```python
from build123d import *

# Parameters (mm, degrees)
SKETCH1_W           = 64
SKETCH1_H           = 42
BOSS_EXTRUDE1_DEPTH = 14.5
FILLET1_R           = 8
FILLET2_R           = 2
SHELL1_T            = -1.6
CUT_EXTRUDE1_REACH  = 70.9
SKETCH2_W           = 3.8
SKETCH2_H           = 24.8
SKETCH3_R           = 3
BOSS_EXTRUDE2_DEPTH = 7.000000018
CUT_EXTRUDE2_REACH  = 77.447
SKETCH4_R           = 1.6
SKETCH5_R           = 4
CUT_EXTRUDE3_DEPTH  = 0.6


with BuildPart() as part:
    # Sketch1 → Boss-Extrude1 (new body)
    with BuildSketch(Plane.XY):
        Rectangle(SKETCH1_W, SKETCH1_H)
    extrude(amount=BOSS_EXTRUDE1_DEPTH)

    # Fillet1
    fillet1_edges = [part.edges().sort_by_distance(p)[0] for p in [
        (-32, 21, 7.25),
        (32, 21, 7.25),
        (32, -21, 7.25),
        (-32, -21, 7.25),
    ]]
    fillet(fillet1_edges, radius=FILLET1_R)

    # Fillet2
    fillet2_edges = [part.edges().sort_by_distance(p)[0] for p in [
        (0, -21, 14.5),
        (-32, 0, 14.5),
        (32, 0, 14.5),
        (0, 21, 14.5),
        (29.656854249, 18.656854249, 14.5),
        (-29.656854249, 18.656854249, 14.5),
        (29.656854249, -18.656854249, 14.5),
        (-29.656854249, -18.656854249, 14.5),
    ]]
    fillet(fillet2_edges, radius=FILLET2_R)

    # Shell1
    shell1_openings = [part.faces().sort_by_distance(p)[0] for p in [
        (0, 0, 0),
    ]]
    offset(amount=SHELL1_T, openings=shell1_openings, kind=Kind.INTERSECTION)

    # Sketch2 → Cut-Extrude1 (cut, up to next)
    with BuildSketch(Plane(origin=(32, 0, 0), x_dir=(0, 0, -1), z_dir=(1, 0, 0)), mode=Mode.PRIVATE) as cut_extrude1_sk1:
        with Locations((-1.9, 0)):
            Rectangle(SKETCH2_W, SKETCH2_H)
    cut_extrude1_tool1 = extrude(cut_extrude1_sk1.sketch, amount=-CUT_EXTRUDE1_REACH, mode=Mode.PRIVATE) & part.part
    add(cut_extrude1_tool1.solids().sort_by_distance((32, 0, 1.9))[0], mode=Mode.SUBTRACT)

    # Sketch3 → Boss-Extrude2 (add)
    with BuildSketch(Plane.ZY.offset(32)):
        with Locations(Location((7, 0, 0), (0, 0, 180))):
            Circle(SKETCH3_R)
    extrude(amount=BOSS_EXTRUDE2_DEPTH)

    # Sketch4 → Cut-Extrude2 (cut, up to next)
    with BuildSketch(Plane.ZY.offset(39.000000018), mode=Mode.PRIVATE) as cut_extrude2_sk1:
        with Locations((7, 0)):
            Circle(SKETCH4_R)
    cut_extrude2_tool1 = extrude(cut_extrude2_sk1.sketch, amount=-CUT_EXTRUDE2_REACH, mode=Mode.PRIVATE) & part.part
    add(cut_extrude2_tool1.solids().sort_by_distance((-39, 0, 7))[0], mode=Mode.SUBTRACT)

    # Sketch5 → Cut-Extrude3 (cut)
    with BuildSketch(Plane.XY.offset(14.5)):
        with Locations((-19, 0)):
            Circle(SKETCH5_R)
    extrude(amount=-CUT_EXTRUDE3_DEPTH, mode=Mode.SUBTRACT)


solid = part.part
```
The model under review builds one solid part; all positions refer to its coordinate system, in mm. A direction names the side the tool comes from. Give positions to 0.01 mm unless a question says otherwise; leave off trailing zeros. Loops run counter-clockwise (first coordinate to the right, second up) from the corner with the lowest first, then second, coordinate; pieces in that order, holes last. Notation, with made-up numbers: (42, 13) - (58, 13) arc R16 ccw to (58, 43) - close; hole circle Ø4 at (85.5, -4.75). An arc over 180 degrees is marked (long way). Answer as a JSON object with one key per item and string values.
Q1. Add section B-B on x = 19. State the section outline as (y, z) points, plus the area to 3 significant figures.
Worked out:
{"outline": "(-21, 0) - (-19.4, 0) - (-19.4, 12.5) arc R0.4 cw to (-19, 12.9) - (19, 12.9) arc R0.4 cw to (19.4, 12.5) - (19.4, 0) - (21, 0) - (21, 12.5) arc R2 ccw to (19, 14.5) - (-19, 14.5) arc R2 ccw to (-21, 12.5) - close", "area": "107 mm^2"}
Q2. Add section A-A on y = 0. State the section outline as (x, z) points, plus the area to 3 significant figures.
Worked out:
{"outline": "(-39, 4) - (-32, 4) - (-32, 0) - (-30.4, 0) - (-30.4, 5.4) - (-39, 5.4) - close; (-39, 8.6) - (-30.4, 8.6) - (-30.4, 12.5) arc R0.4 cw to (-30, 12.9) - (30, 12.9) arc R0.4 cw to (30.4, 12.5) - (30.4, 3.8) - (32, 3.8) - (32, 12.5) arc R2 ccw to (30, 14.5) - (-15, 14.5) - (-15, 13.9) - (-23, 13.9) - (-23, 14.5) - (-30, 14.5) arc R2 ccw to (-32, 12.5) - (-32, 10) - (-39, 10) - close", "area": "146 mm^2"}
Q3. For faces 5 (the flat face through (0, 19.4, 6)), 6 (the flat face through (31, -12.4, 2)), 7 (the flat face through (-19, 0, 13.9)), 8 (the cylindrical face through (-31.4, -0.18, 13.93)), list the 3-axis set-ups (+Z, -Z, +X, -X, +Y, -Y) from which the entire face can be reached by the end or side of a thin tool; tool diameter is ignored.
Worked out:
{"face 5": "-Z", "face 6": "-Z, +X", "face 7": "+Z", "face 8": "+Z, -X, +Y, -Y"}
Q4. To check wall thickness, follow line 1 along Y through (x, z) = (-32.5, 7); line 2 along X through (y, z) = (10, 7.5); line 3 along Y through (x, z) = (-0.5, 8.5). State the ranges of each line that lie inside material, in increasing order.
Worked out:
{"line 1": "y = -3 to -1.6, 1.6 to 3", "line 2": "x = -32 to -30.4, 30.4 to 32", "line 3": "y = -21 to -19.4, 19.4 to 21"}
Q5. Insertion check: pin 1 (5 mm diameter, centred on x = 5.5, y = -10.5, fed in from -Z); pin 2 (0.8 mm diameter, centred on x = 31, z = 2, fed in from +Y); pin 3 (1 mm diameter, centred on y = -8.5, z = 2, fed in from +X). Each pin has a flat end and moves straight along its axis. Give the tip position at first contact, or say it passes through.
Worked out:
{"pin 1": "stops at z = 12.9", "pin 2": "stops at y = 17.52", "pin 3": "stops at x = -30.4"}
Q6. Add section D-D on z = 7. State the section outline as (x, y) points.
Worked out:
{"outline": "(-39, -3) - (-32, -3) - (-32, -13) arc R8 ccw to (-24, -21) - (24, -21) arc R8 ccw to (32, -13) - (32, 13) arc R8 ccw to (24, 21) - (-24, 21) arc R8 ccw to (-32, 13) - (-32, 3) - (-39, 3) - (-39, 1.6) - (-30.4, 1.6) - (-30.4, 13) arc R6.4 cw to (-24, 19.4) - (24, 19.4) arc R6.4 cw to (30.4, 13) - (30.4, -13) arc R6.4 cw to (24, -19.4) - (-24, -19.4) arc R6.4 cw to (-30.4, -13) - (-30.4, -1.6) - (-39, -1.6) - close"}
Q7. Add section C-C on y = -5. State the section outline as (x, z) points.
Worked out:
{"outline": "(-32, 0) - (-30.4, 0) - (-30.4, 12.5) arc R0.4 cw to (-30, 12.9) - (30, 12.9) arc R0.4 cw to (30.4, 12.5) - (30.4, 3.8) - (32, 3.8) - (32, 12.5) arc R2 ccw to (30, 14.5) - (-30, 14.5) arc R2 ccw to (-32, 12.5) - close"}
Q8. Mouldability with a two-part tool opening along Y and no side actions: class faces 1 (the cylindrical face through (29.594, -18.719, 6.338)), 2 (the cylindrical face through (-29.719, 18.594, 6.338)), 3 (the cylindrical face through (-28.57, 17.48, 6.34)), 4 (the flat face through (-30.4, 0, 5)) as +Y half, -Y half, draft (parallel to the pull), parting line (faces both ways), or undercut.
Worked out:
{"face 1": "-Y half", "face 2": "+Y half", "face 3": "undercut", "face 4": "undercut"}
